```python
from build123d import *

# Parameters (mm, degrees)
F1_DEPTH = 20
F3_DEPTH = 17.88954382
F4_W     = 10
F4_H     = 5
F5_DEPTH = 2.501
F7_DEPTH = 30.001


with BuildPart() as f1:
    # F0 (on Front) → F1 (new body)
    with BuildSketch(Plane.XZ):
        Polygon((0, 20), (0, 0), (30, 0), (30, 5), align=None)
    extrude(amount=F1_DEPTH)

    # F2 (on face) → F3 (cut, through all)
    with BuildSketch(Plane(origin=(8, 0, 16), x_dir=(0.894427191, 0, -0.4472135955), z_dir=(0.4472135955, 0, 0.894427191))):
        Polygon((24.5967477525, -15), (24.5967477525, -10), (24.5967477525, -5), (19.5967477525, -5), (19.5967477525, -10), (19.5967477525, -15), align=None)
    extrude(amount=-F3_DEPTH, mode=Mode.SUBTRACT)

    # F4 (on face) → F5 (cut, through all)
    with BuildSketch(Plane.YZ.offset(30)):
        with Locations((-10, 2.5)):
            Rectangle(F4_W, F4_H)
    extrude(amount=-F5_DEPTH, mode=Mode.SUBTRACT)

    # F6 (on face) → F7 (cut, through all)
    with BuildSketch(Plane(origin=(0, 0, 0), x_dir=(0, -1, 0), z_dir=(-1, 0, 0))):
        Polygon((15, 20), (10, 20), (5, 20), (5, 10), (10, 10), (15, 10), align=None)
    extrude(amount=-F7_DEPTH, mode=Mode.SUBTRACT)


solid = f1.part
```
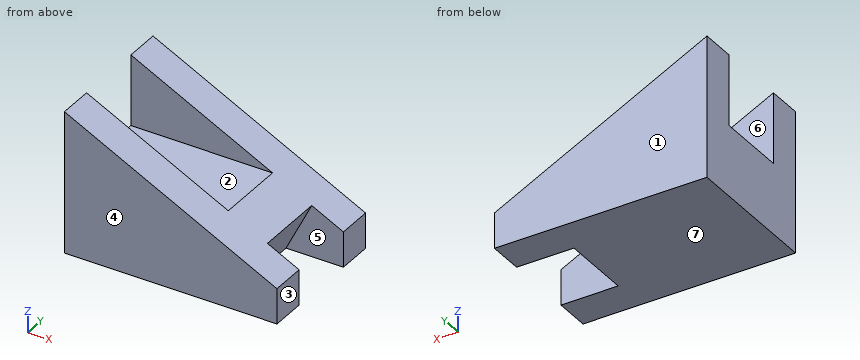
CAD build for the part. Positions are in the model's coordinates, mm. Face numbers are marked on the shaded views. A direction names the side the tool comes from. Round coordinates to 2 decimals unless told otherwise and drop trailing zeros. Order: outer loops, then holes, each group sorted by start corner. A loop starts at its lowest first (then second) coordinate and runs counter-clockwise, first axis right, second up.
Item 1: Probe line 1 along Z through (x, y) = (19.5, -8); line 2 along X through (y, z) = (-18, 13); line 3 along X through (y, z) = (-10.5, 9.75). List the from-to ranges inside material, lowest first.
Item 2: Saw through at A-A on z = 17.25. Write the cut outline in (x, y).
Item 3: Mould opens along Y. For the marked faces 1, 2, 3 and 4 say: pulls with the +Y half, pulls with the -Y half, needs draft (parallel to the pull), parting line crosses it, or undercut.
Item 4: Pin check, flat tip, straight feed: pin 1 (3 mm diameter, centred on x = 10, y = -9.5, fed in from +Z). Stop position of the tip, or through.
Item 5: Saw through at B-B on x = 26. Write the cut outline in (y, z).
Item 6: Saw through at D-D on y = -10.5. Write the cut outline in (x, z), then the cut area to 3 significant figures.
Item 7: Saw through at C-C on x = 3. Write the cut outline in (y, z), then the cut area to 3 significant figures.
Item 8: Tool access for the marked faces 5, 6 and 7: list every direction of +Z, -Z, +X, -X, +Y, -Y with a clear straight run to the whole face (end or side of a thin tool).
Reported:
1. line 1: z = 0 to 10
1. line 2: x = 0 to 14
1. line 3: x = 0 to 20.5
2. outline: (0, -20) - (5.5, -20) - (5.5, -15) - (0, -15) - close; (0, -5) - (5.5, -5) - (5.5, 0) - (0, 0) - close
3. face 1: pulls with the +Y half
3. face 2: undercut
3. face 3: needs draft
3. face 4: pulls with the -Y half
4. pin 1: stops at z = 10
5. outline: (-20, 0) - (-15, 0) - (-15, 7) - (-20, 7) - close; (-5, 0) - (0, 0) - (0, 7) - (-5, 7) - close
6. outline: (0, 0) - (21.91, 0) - (25.53, 7.24) - (20, 10) - (0, 10) - close
6. area: 235 mm2
7. outline: (-20, 0) - (0, 0) - (0, 18.5) - (-5, 18.5) - (-5, 10) - (-15, 10) - (-15, 18.5) - (-20, 18.5) - close
7. area: 285 mm2
8. face 5: -Z, +X
8. face 6: +Z, +X, -X
8. face 7: -Z, +X, -X, +Y, -Y
